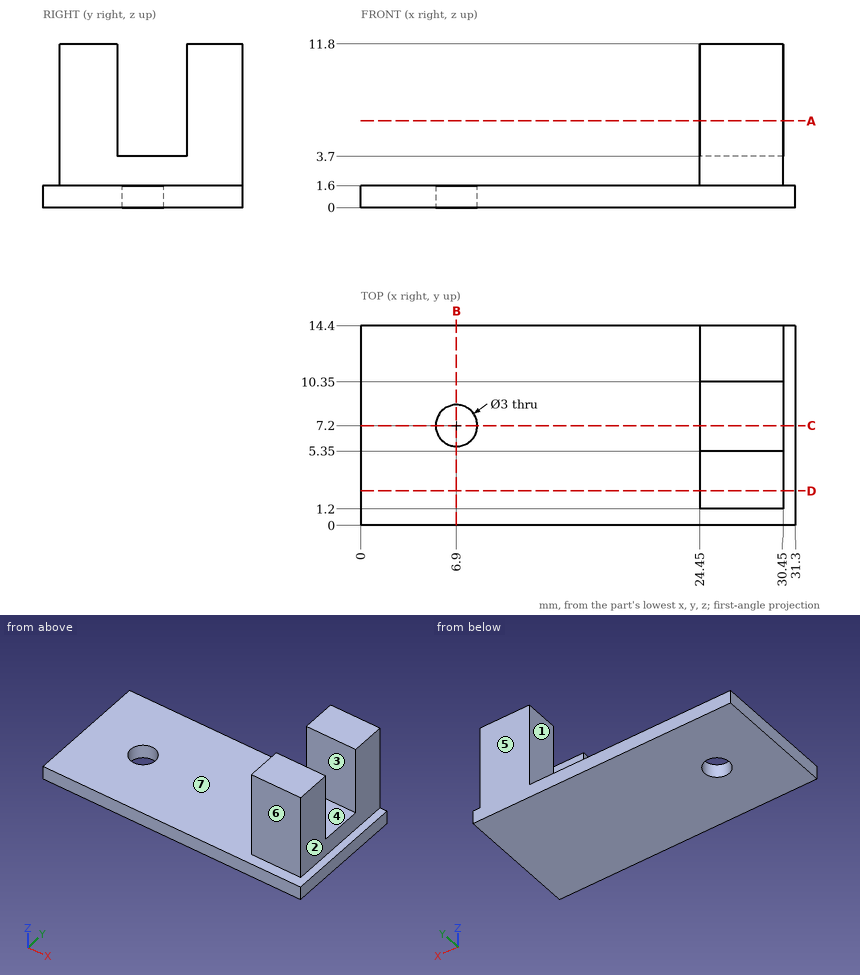
Print and shaded views of the part. All mm, measured from the part's lowest x, y and z. A direction names the side the tool comes from. Coordinates: 2 decimals unless noted, no trailing zeros. Order: outer loops, then holes, each group sorted by start corner. A loop starts at its lowest first (then second) coordinate and runs counter-clockwise, first axis right, second up. Notation, with made-up numbers: (-18, 56.5) -> (-13, 56.5) arc R26 ccw to (-13, 74.5) -> close; hole circle Ø8 at (69.25, -40). An arc over 180 degrees is marked (long way). Use one line per item in the form item = value. Start each with the question number.
1) Tool access for the marked faces 1, 2 and 3: list every direction of +Z, -Z, +X, -X, +Y, -Y with a clear straight run to the whole face (end or side of a thin tool).
2) Band-saw the part on C-C on y = 7.2. Give the cut face in (x, z), then the cut area to 3 significant figures.
3) Band-saw the part on D-D on y = 2.5. Give the cut face in (x, z), then the cut area to 3 significant figures.
4) Pull direction Y, two halves, no side cores. Call the marked faces 4, 5, 6 and 7: +Y half, -Y half, draft (parallel to the pull), parting line (faces both ways), or undercut.
5) Band-saw the part on B-B on x = 6.9. Give the cut face in (y, z), then the cut area to 3 significant figures.
6) Band-saw the part on A-A on z = 6.25. Give the cut face in (x, y), then the cut area to 3 significant figures.
7) Drill centre lines: L1, parallel to Y at x = 27.5, z = 10; L2, parallel to Y at x = 6.9, z = 1.2; L3, parallel to Z at x = 22, y = 10.75. Where is each one in solid material? Low to high. Write a range as [from, to].
8) Drop flat-ended pins along their axis: pin 1 (3 mm diameter, centred on y = 10.5, z = 6.5, fed in from -X); pin 2 (1 mm diameter, centred on x = 22, y = 11.5, fed in from +Z); pin 3 (1.5 mm diameter, centred on y = 7, z = 5.5, fed in from +X); pin 4 (1.8 mm diameter, centred on x = 26.5, z = 5.5, fed in from -Y). Give the stop position or say it passes through.
Entries:
q1.face_1 = +Z, -X, +Y, -Y
q1.face_2 = +Z, +X, +Y, -Y
q1.face_3 = +Z, +X, -X
q2.outline = (0, 0) -> (5.4, 0) -> (5.4, 1.6) -> (0, 1.6) -> close; (8.4, 0) -> (31.3, 0) -> (31.3, 1.6) -> (30.45, 1.6) -> (30.45, 3.7) -> (24.45, 3.7) -> (24.45, 1.6) -> (8.4, 1.6) -> close
q2.area = 57.9 mm2
q3.outline = (0, 0) -> (31.3, 0) -> (31.3, 1.6) -> (30.45, 1.6) -> (30.45, 11.8) -> (24.45, 11.8) -> (24.45, 1.6) -> (0, 1.6) -> close
q3.area = 111 mm2
q4.face_4 = undercut
q4.face_5 = +Y half
q4.face_6 = -Y half
q4.face_7 = draft
q5.outline = (0, 0) -> (5.7, 0) -> (5.7, 1.6) -> (0, 1.6) -> close; (8.7, 0) -> (14.4, 0) -> (14.4, 1.6) -> (8.7, 1.6) -> close
q5.area = 18.2 mm2
q6.outline = (24.45, 1.2) -> (30.45, 1.2) -> (30.45, 5.35) -> (24.45, 5.35) -> close; (24.45, 10.35) -> (30.45, 10.35) -> (30.45, 14.4) -> (24.45, 14.4) -> close
q6.area = 49.2 mm2
q7.L1 = [1.2, 5.35], [10.35, 14.4]
q7.L2 = [0, 5.7], [8.7, 14.4]
q7.L3 = [0, 1.6]
q8.pin_1 = 24.45
q8.pin_2 = 1.6
q8.pin_3 = through
q8.pin_4 = 1.2
